```python
from build123d import *

# Parameters (mm, degrees)
F0_W     = 762
F0_H     = 76.2
F0_R     = 12.7
F1_DEPTH = 6.35
F2_W     = 9.525
F2_H     = 50.8
F3_DEPTH = 25.4
F4_R     = 12.7
F5_R     = 1.6002


with BuildPart() as f1:
    # F0 (on Front) → F1 (new body)
    with BuildSketch(Plane.XZ):
        with Locations((190.5, -15.812627)):
            Rectangle(F0_W, F0_H)
        with Locations((-127, -15.812627)):
            Circle(F0_R, mode=Mode.SUBTRACT)
        with Locations((0, -15.812627)):
            Circle(F0_R, mode=Mode.SUBTRACT)
        with Locations((127, -15.812627)):
            Circle(F0_R, mode=Mode.SUBTRACT)
        with Locations((254, -15.812627)):
            Circle(F0_R, mode=Mode.SUBTRACT)
        with Locations((381, -15.812627)):
            Circle(F0_R, mode=Mode.SUBTRACT)
        with Locations((508, -15.812627)):
            Circle(F0_R, mode=Mode.SUBTRACT)
    extrude(amount=F1_DEPTH)

    # F2 (on face) → F3 (cut)
    with BuildSketch(Plane.XZ.offset(6.35)):
        with Locations((34.9377, -15.812627)):
            Rectangle(F2_W, F2_H)
        with Locations((47.6377, -15.812627)):
            Rectangle(F2_W, F2_H)
        with Locations((60.3377, -15.812627)):
            Rectangle(F2_W, F2_H)
        with Locations((73.0377, -15.812627)):
            Rectangle(F2_W, F2_H)
        with Locations((85.7377, -15.812627)):
            Rectangle(F2_W, F2_H)
        with Locations((161.9377, -15.812627)):
            Rectangle(F2_W, F2_H)
        with Locations((174.6377, -15.812627)):
            Rectangle(F2_W, F2_H)
        with Locations((187.3377, -15.812627)):
            Rectangle(F2_W, F2_H)
        with Locations((200.0377, -15.812627)):
            Rectangle(F2_W, F2_H)
        with Locations((212.7377, -15.812627)):
            Rectangle(F2_W, F2_H)
        with Locations((288.9377, -15.812627)):
            Rectangle(F2_W, F2_H)
        with Locations((301.6377, -15.812627)):
            Rectangle(F2_W, F2_H)
        with Locations((314.3377, -15.812627)):
            Rectangle(F2_W, F2_H)
        with Locations((327.0377, -15.812627)):
            Rectangle(F2_W, F2_H)
        with Locations((339.7377, -15.812627)):
            Rectangle(F2_W, F2_H)
        with Locations((415.9377, -15.812627)):
            Rectangle(F2_W, F2_H)
        with Locations((428.6377, -15.812627)):
            Rectangle(F2_W, F2_H)
        with Locations((441.3377, -15.812627)):
            Rectangle(F2_W, F2_H)
        with Locations((454.0377, -15.812627)):
            Rectangle(F2_W, F2_H)
        with Locations((466.7377, -15.812627)):
            Rectangle(F2_W, F2_H)
        with Locations((-81.209007, -15.812627)):
            Rectangle(F2_W, F2_H)
        with Locations((-68.509007, -15.812627)):
            Rectangle(F2_W, F2_H)
        with Locations((-55.809007, -15.812627)):
            Rectangle(F2_W, F2_H)
        with Locations((-43.109007, -15.812627)):
            Rectangle(F2_W, F2_H)
        with Locations((-30.409007, -15.812627)):
            Rectangle(F2_W, F2_H)
    extrude(amount=-F3_DEPTH, mode=Mode.SUBTRACT)

    # F4
    f4_edges = [f1.edges().sort_by_distance(p)[0] for p in [
        (-190.5, -3.175, 22.287373),
        (-190.5, -3.175, -53.912627),
        (571.5, -3.175, 22.287373),
        (571.5, -3.175, -53.912627),
    ]]
    fillet(f4_edges, radius=F4_R)

    # F5
    f5_edges = [f1.edges().sort_by_distance(p)[0] for p in [
        (190.5, -6.35, 22.287373),
        (190.5, 0, 22.287373),
    ]]
    fillet(f5_edges, radius=F5_R)


solid = f1.part
```
Verification items for the finished model (mm, model axes). Round coordinates to 2 decimals unless told otherwise and drop trailing zeros. Order: outer loops, then holes, each group sorted by start corner. A loop starts at its lowest first (then second) coordinate and runs counter-clockwise, first axis right, second up.
1) Cross-section at B-B, the plane x = 251.5. Record the cut outline in (y, z), plus the area to 3 significant figures.
Geometry says:
outline: (-6.35, -52.31) arc R1.6 ccw to (-4.75, -53.91) - (-1.6, -53.91) arc R1.6 ccw to (0, -52.31) - (0, -28.26) - (-6.35, -28.26) - close; (-6.35, -3.36) - (0, -3.36) - (0, 20.69) arc R1.6 ccw to (-1.6, 22.29) - (-4.75, 22.29) arc R1.6 ccw to (-6.35, 20.69) - close
area: 324 mm2
2) Draft check along X on faces 1 (the cylindrical face through (132.86, -3.13, -27.08)), 2 (the flat face through (185, 0, -48)), 3 (the cylindrical face through (567.681, -3.197, 18.666)). Enter one of: +X half, -X half, draft (parallel to the pull), parting line (faces both ways), or undercut.
Geometry says:
face 1: undercut
face 2: draft
face 3: +X half
3) Cross-section at C-C, the plane y = -3.25. Give the number of separate pieces and of enclosed holes in the cut face, plus the area to 3 significant figures.
Geometry says:
separate pieces: 1
enclosed holes: 31
area: 42,800 mm2
4) Material ranges on line 1 (Z direction, x = 508, y = -4); line 2 (Z direction, x = 59, y = -1.5); line 3 (X direction, y = -1.5, z = 11), recorded low to high.
Geometry says:
line 1: z = -53.91 to -28.51, -3.11 to 22.29
line 2: z = -53.91 to -41.21, 9.59 to 22.28
line 3: x = -190.42 to 571.42
5) Cross-section at A-A, the plane x = -127. Record the cut outline in (y, z), plus the area to 3 significant figures.
Geometry says:
outline: (-6.35, -52.31) arc R1.6 ccw to (-4.75, -53.91) - (-1.6, -53.91) arc R1.6 ccw to (0, -52.31) - (0, -28.51) - (-6.35, -28.51) - close; (-6.35, -3.11) - (0, -3.11) - (0, 20.69) arc R1.6 ccw to (-1.6, 22.29) - (-4.75, 22.29) arc R1.6 ccw to (-6.35, 20.69) - close
area: 320 mm2
